Answer from the drawing. Dimensions are ordinates in mm from the lowest x, y and z of the part. A direction names the side the tool comes from. Round coordinates to 2 decimals unless told otherwise and drop trailing zeros. Write each loop counter-clockwise with the first axis right and the second up, starting at its lowest first coordinate (ties: lowest second). Pieces come first, ordered by that corner, then holes. Notation, with made-up numbers: (87, -30) -> (136, -30) arc R5 ccw to (136, -23) -> close; hole circle Ø1 at (65.5, 38.5). An arc over 180 degrees is marked (long way). Return JSON: item names as keys, results as strings. Group by question number.
(1) A cutting plane is placed at A-A on z = 1.85. State how many separate pieces and enclosed holes the cut face has.
(2) For the marked faces 1, 2 and 3, determine the directions among +Z, -Z, +X, -X, +Y, -Y from which every point of the face is accessible in a straight line to the end or side of a thin tool.
(3) A cutting plane is placed at C-C on x = 9. Give the vertices of the cut face in (y, z) (1 decimal).
(4) Given pin 1 (5.5 mm diameter, centred on x = 19.05, y = 56.04, fed in from +Z) (3 decimals); pin 2 (1 mm diameter, centred on y = 32, z = 1, fed in from -X); pin 3 (1 mm diameter, centred on y = 46, z = 2.5, fed in from +X), each flat-ended and moving along its own axis, determine where each tip first touches the part or whether it passes through.
(5) A cutting plane is placed at B-B on y = 40.5. Give the vertices of the cut face in (x, z) (1 decimal).
(6) The mould has two halves that part along X. Classify the marked faces 4, 5 and 6: released by +X, released by -X, zero draft, split by the parting line, or undercut.
(7) Straight lines are drawn through the part: line 1 (Y direction, x = 20.5, z = 1) (1 decimal); line 2 (X direction, y = 42, z = 0.4); line 3 (Y direction, x = 7, z = 1.95) (1 decimal). For each, find the intervals that lie inside material, in ascending order.
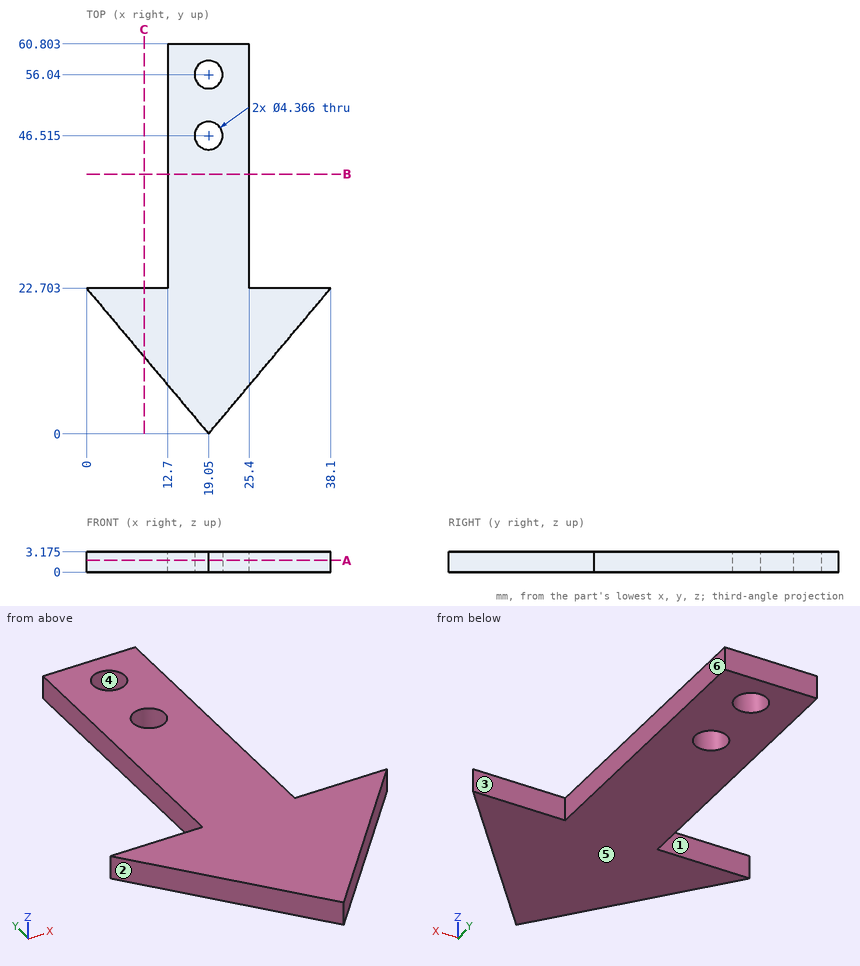
Checks:
{
 "1": {"separate pieces": "1", "enclosed holes": "2"},
 "2": {"face 1": "+Z, -Z, -X, +Y", "face 2": "+Z, -Z, -X, -Y", "face 3": "+Z, -Z, +X, +Y"},
 "3": {"outline": "(12, 0) -> (22.7, 0) -> (22.7, 3.2) -> (12, 3.2) -> close"},
 "4": {"pin 1": "stops at z = 3.175", "pin 2": "stops at x = 12.7", "pin 3": "stops at x = 25.4"},
 "5": {"outline": "(12.7, 0) -> (25.4, 0) -> (25.4, 3.2) -> (12.7, 3.2) -> close"},
 "6": {"face 4": "undercut", "face 5": "zero draft", "face 6": "released by +X"},
 "7": {"line 1": "y = 1.7 to 44.9, 48.1 to 54.4, 57.7 to 60.8", "line 2": "x = 12.7 to 25.4", "line 3": "y = 14.4 to 22.7"}
}
